CAD build for the part. Positions are in the model's coordinates, mm. A direction names the side the tool comes from. Coordinates: 2 decimals unless noted, no trailing zeros. Order: outer loops, then holes, each group sorted by start corner. A loop starts at its lowest first (then second) coordinate and runs counter-clockwise, first axis right, second up. Notation, with made-up numbers: M 2.25,0.25 L 15.25,0.25 A28 ccw 15.25,31.25 Z; hole C -16.5,68 d7. An arc over 180 degrees is marked long. One line per item, written item: value.
from build123d import *

# Parameters (mm, degrees)
F1_DEPTH = 609.6
F2_R     = 4.7625
F3_DEPTH = 25.4


with BuildPart() as f1:
    # F0 (on Front) → F1 (new body)
    with BuildSketch(Plane.XZ):
        with BuildLine():
            Line((-9.921028, -11.871202), (9.128972, -11.871202))
            ThreePointArc((9.128972, -11.871202), (11.374036, -10.941266), (12.303972, -8.696202))
            Line((12.303972, -8.696202), (12.303972, 10.353798))
            ThreePointArc((12.303972, 10.353798), (11.374036, 12.598862), (9.128972, 13.528798))
            Line((9.128972, 13.528798), (-9.921028, 13.528798))
            ThreePointArc((-9.921028, 13.528798), (-12.166092, 12.598862), (-13.096028, 10.353798))
            Line((-13.096028, 10.353798), (-13.096028, -8.696202))
            ThreePointArc((-13.096028, -8.696202), (-12.166092, -10.941266), (-9.921028, -11.871202))
        make_face()
        with BuildLine():
            ThreePointArc((9.128972, -5.521202), (8.199036, -7.766266), (5.953972, -8.696202))
            Line((5.953972, -8.696202), (-6.746028, -8.696202))
            ThreePointArc((-6.746028, -8.696202), (-8.991092, -7.766266), (-9.921028, -5.521202))
            Line((-9.921028, -5.521202), (-9.921028, 7.178798))
            ThreePointArc((-9.921028, 7.178798), (-8.991092, 9.423862), (-6.746028, 10.353798))
            Line((-6.746028, 10.353798), (5.953972, 10.353798))
            ThreePointArc((5.953972, 10.353798), (8.199036, 9.423862), (9.128972, 7.178798))
            Line((9.128972, 7.178798), (9.128972, -5.521202))
        make_face(mode=Mode.SUBTRACT)
    extrude(amount=F1_DEPTH)

    # F2 (on face) → F3 (cut)
    with BuildSketch(Plane.YZ.offset(12.303972)):
        with Locations((-228.6, 0.828798)):
            Circle(F2_R)
        with Locations((-127, 0.828798)):
            Circle(F2_R)
    extrude(amount=-F3_DEPTH, mode=Mode.SUBTRACT)


solid = f1.part
Q1. Pin check, flat tip, straight feed: pin 1 Ø12 at (x, z) = (-2, 0.5) entering from +Y. Stop position of the tip, or through.
Recorded:
pin 1: passes through
Q2. Mould opens along X. For faces 1 (the face through (9.129, -301, 1)), 2 (the face through (0, -301, 13.529)), 3 (the face through (12.304, -301, 1)) say: released by +X, released by -X, zero draft, split by the parting line, or undercut.
Recorded:
face 1: undercut
face 2: zero draft
face 3: released by +X
Q3. Which spindle directions (+Z, -Z, +X, -X, +Y, -Y) get a long thin tool onto all of the face, cutting with end or side? Do faces 4 (the face through (0, -301, 10.354)), 5 (the face through (-13.096, -301, 1)). Say none if no direction does.
Recorded:
face 4: +Y, -Y
face 5: +Z, -Z, -X, +Y, -Y
Q4. Slice it at B-B (y = -310.5). List the corners of the cut face in (x, z) (3 decimals).
Recorded:
outline: M -13.096,-8.696 A3.175 ccw -9.921,-11.871 L 9.129,-11.871 A3.175 ccw 12.304,-8.696 L 12.304,10.354 A3.175 ccw 9.129,13.529 L -9.921,13.529 A3.175 ccw -13.096,10.354 Z; hole M -9.921,-5.521 A3.175 ccw -6.746,-8.696 L 5.954,-8.696 A3.175 ccw 9.129,-5.521 L 9.129,7.179 A3.175 ccw 5.954,10.354 L -6.746,10.354 A3.175 ccw -9.921,7.179 Z
Q5. Drill centre lines: line 1 along X through (y, z) = (-326, 2); line 2 along Z through (x, y) = (-4.75, -274.5); line 3 along X through (y, z) = (-261, 8). Where is each one in solid material? Low to high.
Recorded:
line 1: x = -13.1 to -9.92, 9.13 to 12.3
line 2: z = -11.87 to -8.7, 10.35 to 13.53
line 3: x = -13.1 to -9.81, 9.02 to 12.3
Q6. Slice it at A-A (x = 1.5). List the corners of the cut face in (y, z).
Recorded:
outline: M -609.6,-11.87 L 0,-11.87 L 0,-8.7 L -609.6,-8.7 Z; M -609.6,10.35 L 0,10.35 L 0,13.53 L -609.6,13.53 Z
